Answer from the drawing. Dimensions are ordinates in mm from the lowest x, y and z of the part. A direction names the side the tool comes from. Give positions to 0.01 mm unless a question says otherwise; leave off trailing zeros. Loops run counter-clockwise (first coordinate to the right, second up) from the corner with the lowest first, then second, coordinate; pieces in that order, holes last.
Item 1: Each of these flat-tipped pins is pushed along its axis until it touches: pin 1 Ø6.5 at (y, z) = (22, 41.5) entering from +X; pin 2 Ø0.9 at (x, z) = (1.5, 22) entering from +Y; pin 3 Ø8 at (x, z) = (30.5, 51) entering from +Y. Where does it stop, or does it pass through?
Item 2: Section B-B, the plane x = 29.5 is taken. Give the vertices of the cut face in (y, z), and give its area (3 significant figures).
Item 3: Section D-D, the plane z = 8.5 is taken. Give the vertices of the cut face in (x, y).
Item 4: A tool of negligible diameter and unlimited length cuts with its end or side. For the marked faces 1 and 2, from which of +Z, -Z, +X, -X, +Y, -Y can it reach the whole face along a straight path? Write none if from no direction.
Item 5: Consider line 1 along Y through (x, z) = (0.8, 8.5); line 2 along Y through (x, z) = (1.65, 135); line 3 along X through (y, z) = (20.5, 124). Determine where each line is inside the solid, lowest interval first.
Item 6: Section A-A, the plane z = 80 is taken. Give the vertices of the cut face in (x, y).
Item 7: Section C-C, the plane y = 22 is taken. Give the number of separate pieces and of enclosed holes in the cut face, and give its area (3 significant figures).
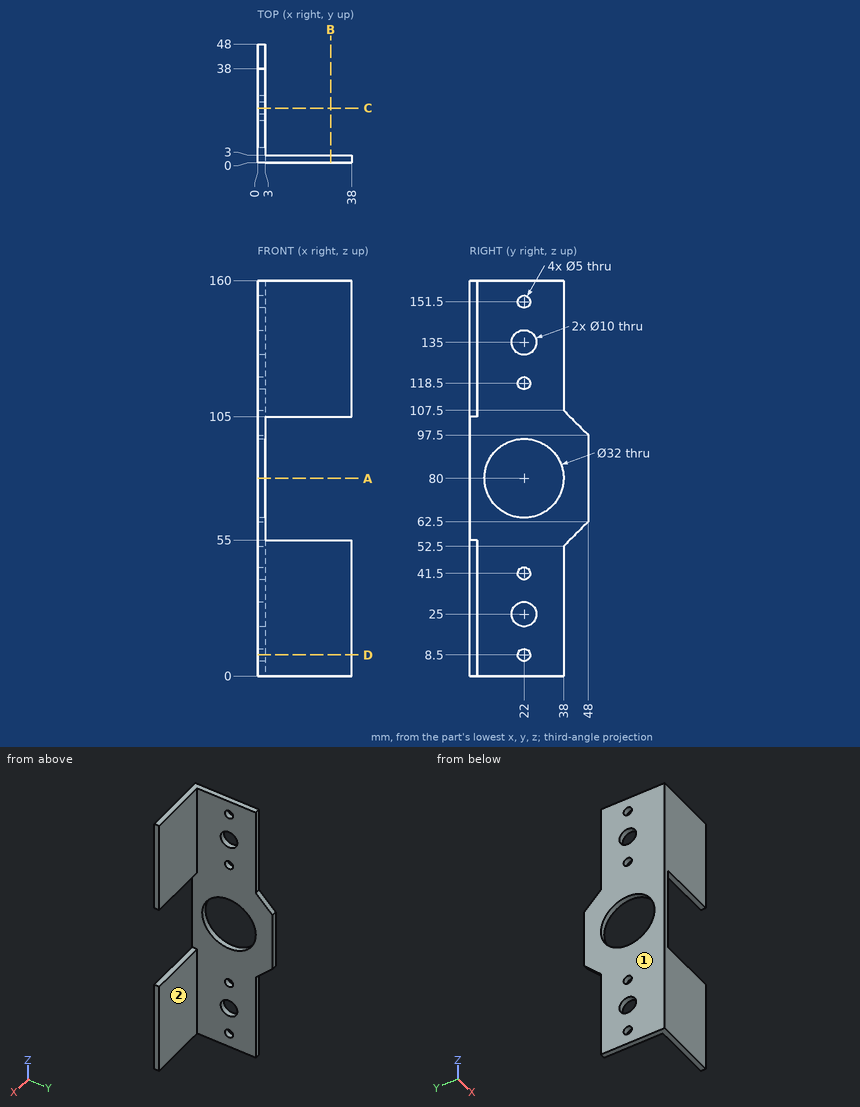
Worked answers:
1. pin 1: stops at x = 3
1. pin 2: stops at y = 38
1. pin 3: stops at y = 3
2. outline: (0, 0) - (3, 0) - (3, 55) - (0, 55) - close; (0, 105) - (3, 105) - (3, 160) - (0, 160) - close
2. area: 330 mm2
3. outline: (0, 0) - (38, 0) - (38, 3) - (3, 3) - (3, 19.5) - (0, 19.5) - close; (0, 24.5) - (3, 24.5) - (3, 38) - (0, 38) - close
4. face 1: +Z, -Z, -X, +Y, -Y
4. face 2: +Z, -Z, +X, +Y
5. line 1: y = 0 to 19.5, 24.5 to 38
5. line 2: y = 0 to 17, 27 to 38
5. line 3: x = 0 to 3
6. outline: (0, 0) - (3, 0) - (3, 6) - (0, 6) - close; (0, 38) - (3, 38) - (3, 48) - (0, 48) - close
7. separate pieces: 8
7. enclosed holes: 0
7. area: 264 mm2
